Answer from the drawing. Dimensions are ordinates in mm from the lowest x, y and z of the part. Coordinates: 2 decimals unless noted, no trailing zeros. Write each loop counter-clockwise with the first axis right and the second up, starting at its lowest first coordinate (ties: lowest second). Pieces come first, ordered by that corner, then holes.
(1) The part is cut by section A-A, the plane y = 3.75. Determine the outline of the cut face in (x, z).
(2) Straight lines are drawn through the part: line 1 along X through (y, z) = (2, 67.15); line 2 along X through (y, z) = (5, 67.15); line 3 along X through (y, z) = (1, 35). For each, find the intervals that lie inside material, in ascending order.
(3) Given pin 1 (2 mm diameter, centred on x = 76, y = 5.5, fed in from -Z); pin 2 (2 mm diameter, centred on x = 56.5, y = 7, fed in from +Z); pin 3 (6 mm diameter, centred on x = 116, z = 24.5, fed in from +Y); pin 4 (6 mm diameter, centred on x = 66.5, z = 113, fed in from -Y), each flat-ended and moving along its own axis, determine where each tip first touches the part or whether it passes through.
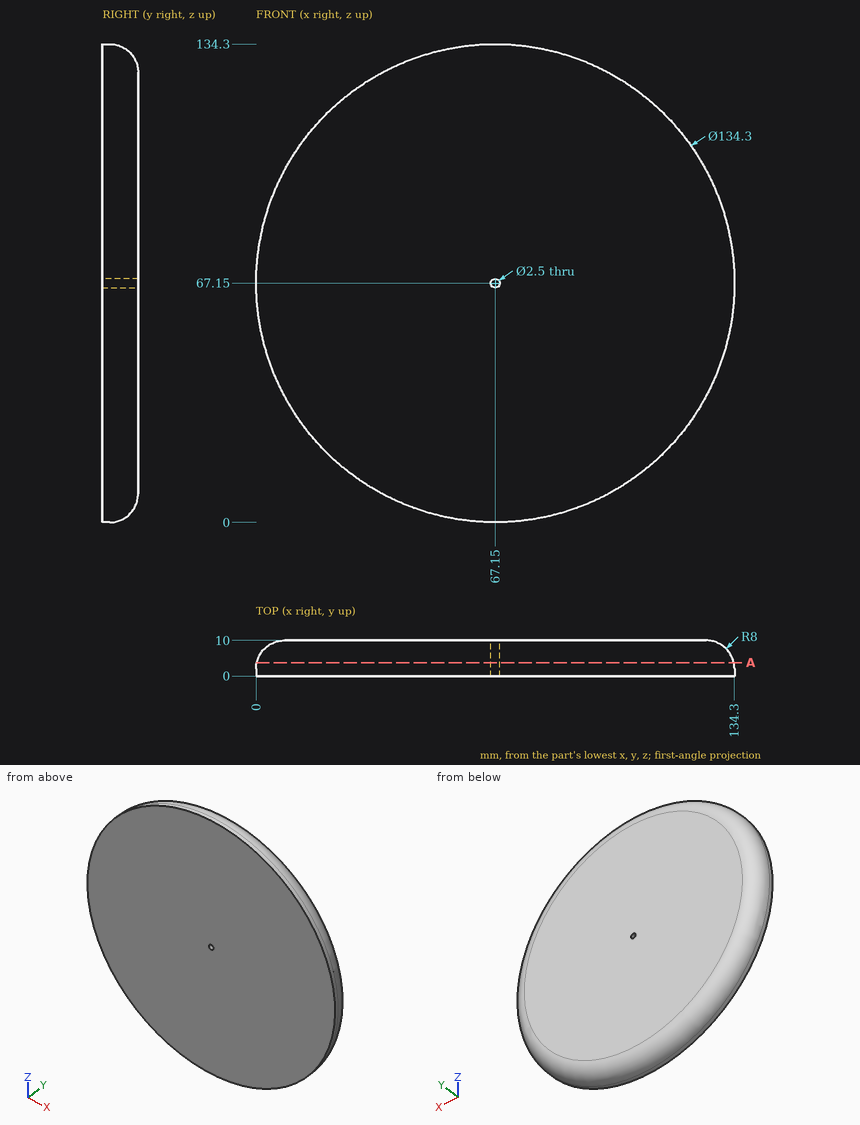
Computed:
1. outline: circle Ø133.91 at (67.15, 67.15); hole circle Ø2.5 at (67.15, 67.15)
2. line 1: x = 0 to 65.9, 68.4 to 134.3
2. line 2: x = 0.58 to 65.9, 68.4 to 133.72
2. line 3: x = 8.2 to 126.1
3. pin 1: stops at z = 0.97
3. pin 2: stops at z = 132.39
3. pin 3: stops at y = 9.53
3. pin 4: stops at y = 0
